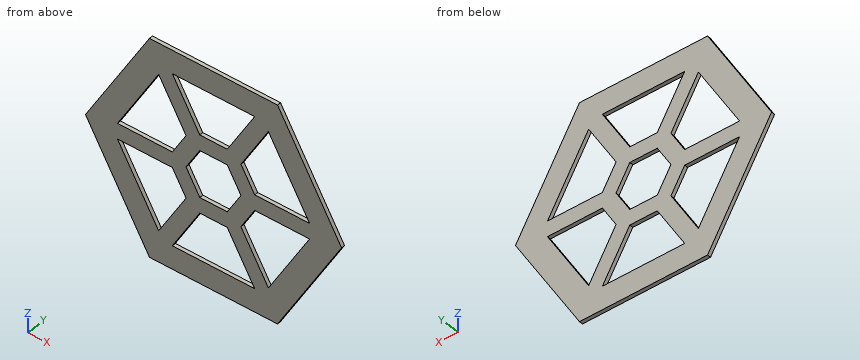
Autodesk Inventor part; units mm, degrees
ref_plane "YZ Plane" through (0, 0, 0) normal (1, 0, 0) x (0, 1, 0)
ref_plane "XZ Plane" through (0, 0, 0) normal (0, 1, 0) x (-1, 0, 0)
ref_plane "XY Plane" through (0, 0, 0) normal (0, 0, 1) x (1, 0, 0)
sketch "Sketch6" plane through (0, 0, 0) normal (0, 1, 0) x (-1, 0, 0)
  circle A0 centre (32.5, -48.5) radius 70
  line L0 (102.5, -48.5) -> (67.5, -109.1218)
  line L1 (67.5, -109.1218) -> (-2.5, -109.1218)
  line L2 (-2.5, -109.1218) -> (-37.5, -48.5)
  line L3 (-37.5, -48.5) -> (-2.5, 12.1218)
  line L4 (-2.5, 12.1218) -> (67.5, 12.1218)
  line L5 (67.5, 12.1218) -> (102.5, -48.5)
  line L6 (32.5, 12.1218) -> (47.5, 12.1218)
  line L7 (47.5, 12.1218) -> (47.5, 5.6218)
  line L8 (47.5, 5.6218) -> (17.5, 5.6218)
  line L9 (17.5, 5.6218) -> (17.5, 12.1218)
  line L10 (47.5, 5.6218) -> (56.6924, 5.6218) construction
  line L11 (17.5, 8.8718) -> (20, 8.8718)
  line L12 (47.5, 8.8718) -> (45, 8.8718)
  line L13 (45, 8.8718) -> (45, 10.1218)
  line L14 (45, 10.1218) -> (20, 10.1218)
  line L15 (20, 10.1218) -> (20, 7.6218)
  line L16 (20, 7.6218) -> (45, 7.6218)
  line L17 (45, 7.6218) -> (45, 10.1218)
  line L18 (47.5, 5.6218) -> (56.6924, 5.6218)
  line L19 (17.5, 5.6218) -> (11, 5.6218)
  line L20 (17.5, 12.1218) -> (11, 5.6218)
  line L21 (17.5, 12.1218) -> (26.6924, 12.1218) construction
  line L22 (47.5, 12.1218) -> (54, 5.6218)
  line L23 (85, -18.1891) -> (77.5, -5.1987)
  line L24 (77.5, -5.1987) -> (71.8708, -8.4487)
  line L25 (71.8708, -8.4487) -> (86.8708, -34.4295)
  line L26 (86.8708, -34.4295) -> (92.5, -31.1795)
  line L27 (71.8708, -8.4487) -> (67.2746, -0.4879) construction
  line L28 (89.6854, -32.8045) -> (88.4354, -30.6394)
  line L29 (74.6854, -6.8237) -> (75.9354, -8.9888)
  line L30 (75.9354, -8.9888) -> (77.0179, -8.3638)
  line L31 (77.0179, -8.3638) -> (89.5179, -30.0144)
  line L32 (89.5179, -30.0144) -> (87.3529, -31.2644)
  line L33 (87.3529, -31.2644) -> (74.8529, -9.6138)
  line L34 (74.8529, -9.6138) -> (77.0179, -8.3638)
  line L35 (71.8708, -8.4487) -> (67.2746, -0.4879)
  line L36 (86.8708, -34.4295) -> (90.1208, -40.0587)
  line L37 (92.5, -31.1795) -> (90.1208, -40.0587)
  line L38 (92.5, -31.1795) -> (87.9038, -23.2187) construction
  line L39 (77.5, -5.1987) -> (68.6208, -2.8196)
  line L40 (71.8708, -88.5513) -> (67.2746, -96.5121) construction
  line L41 (74.6854, -90.1763) -> (75.9354, -88.0112)
  line L42 (74.8529, -87.3862) -> (77.0179, -88.6362)
  line L43 (77.5, -91.8013) -> (71.8708, -88.5513)
  line L44 (77.5, -91.8013) -> (68.6208, -94.1804)
  line L45 (71.8708, -88.5513) -> (67.2746, -96.5121)
  line L46 (77.0179, -88.6362) -> (89.5179, -66.9856)
  line L47 (87.3529, -65.7356) -> (74.8529, -87.3862)
  line L48 (71.8708, -88.5513) -> (86.8708, -62.5705)
  line L49 (89.5179, -66.9856) -> (87.3529, -65.7356)
  line L50 (89.6854, -64.1955) -> (88.4354, -66.3606)
  line L51 (86.8708, -62.5705) -> (92.5, -65.8205)
  line L52 (86.8708, -62.5705) -> (90.1208, -56.9413)
  line L53 (92.5, -65.8205) -> (90.1208, -56.9413)
  line L54 (94.9944, -48.5) -> (63.7472, -102.6218)
  line L55 (63.7472, -102.6218) -> (1.2528, -102.6218)
  line L56 (1.2528, -102.6218) -> (-29.9944, -48.5)
  line L57 (-29.9944, -48.5) -> (1.2528, 5.6218)
  line L58 (1.2528, 5.6218) -> (63.7472, 5.6218)
  line L59 (63.7472, 5.6218) -> (94.9944, -48.5)
  line L60 (74.8529, -87.3862) -> (73.1208, -86.3862)
  line L61 (87.3529, -65.7356) -> (85.6208, -64.7356)
  line L62 (87.3529, -31.2644) -> (85.6208, -32.2644)
  line L63 (74.8529, -9.6138) -> (73.1208, -10.6138)
  line L64 (45, 7.6218) -> (45, 5.6218)
  line L65 (20, 7.6218) -> (20, 5.6218)
  line L66 (-29.9944, -48.5) -> (-22.9944, -48.5)
  line L67 (-29.9944, -48.5) -> (-28.2944, -48.5)
  line L68 (-28.2944, -48.5) -> (-22.9944, -48.5)
  circle A1 centre (-26.9944, -48.5) radius 1.5
  line L69 (-29.9944, -48.5) -> (-23.9944, -48.5)
  line L70 (-23.9944, -48.5) -> (-26.9944, -53.6962)
  line L71 (-23.9944, -48.5) -> (-26.9944, -43.3038)
  point P0 (-27.5473, -52.7386)
  point P1 (-28.2775, -45.5261)
  point P2 (88.4354, -30.6394)
  point P3 (75.9354, -8.9888)
  point P4 (76.4767, -8.6763)
  point P5 (89.6854, -32.8045)
  point P6 (86.4869, -65.2356)
  point P7 (88.4354, -66.3606)
  dimension "d127" = 140
  dimension "d87" = 15
  dimension "d88" = 6.5
  dimension "d91" = 2.5
  dimension "d92" = 2.5
  dimension "d95" = 1.25
  dimension "d96" = 25
  dimension "d97" = 2.5
  dimension "d98" = 25
  dimension "d99" = 135
  dimension "d100" = 0
  dimension "d114" = 1.7
  dimension "d117" = 3
  dimension "d121" = 3
  dimension "d123" = 6
  dimension "d128" = 5.1962
  dimension "d129" = 5.1962
  dimension "d130" = 3
extrude "Fronte" add sketch "Sketch6" along normal blind 2 contours L0 L53 L54 L59 L37 L5 | L5 L39 L35 L59 L58 L18 L22 L4 | L1 L2 L3 L4 L20 L58 L57 L56 L55 L54 L45 L44 L0 | L0 L43 L41 L42 L46 L49 L50 L51 | L51 L52 L53 | L26 L28 L32 L31 L30 L29 L24 L5 | L37 L36 L26 | L7 L12 L13 L14 L15 L11 L9 L4 | L22 L18 L7 | L24 L35 L39 | L44 L45 L43 | L50 L49 L61 L48 L51 | L52 L48 L45 L54 L55 L56 L70 L71 L57 L58 L19 L8 L18 L59 L35 L25 L36 | L26 L25 L62 L32 L28 | L9 L19 L20 | L7 L8 L64 L17 L12 | L29 L34 L63 L25 L24 | L43 L48 L60 L42 L41 | L49 L46 L42 L47 | L32 L33 L34 L30 L31 | L11 L15 L65 L8 L9 | L17 L16 L15 L14 L13 | L47 L60 L48 L61 | L25 L63 L33 L62 | L8 L65 L16 L64 | L71 L66 A1 L57 | L66 A1 L70 L56 | A1 L66 | L66 A1
sketch "Sketch11" plane through (0, 0, 0) normal (0, -1, 0) x (1, 0, 0)
  line L0 (-63.7472, 5.6218) -> (-1.2528, -102.6218)
  line L1 (-94.9944, -48.5) -> (29.9944, -48.5)
  line L2 (-63.7472, -102.6218) -> (-1.2528, 5.6218)
  line L3 (-1.2528, 5.6218) -> (-1.2528, -102.6218)
  circle A0 centre (-32.5, -48.5) radius 55
  line L4 (-5, -0.8686) -> (22.5, -48.5)
  line L5 (22.5, -48.5) -> (-5, -96.1314)
  line L6 (-5, -96.1314) -> (-60, -96.1314)
  line L7 (-60, -96.1314) -> (-87.5, -48.5)
  line L8 (-87.5, -48.5) -> (-60, -0.8686)
  line L9 (-60, -0.8686) -> (-5, -0.8686)
  circle A1 centre (-32.5, -48.5) radius 25
  circle A2 centre (-32.5, -48.5) radius 15
  line L10 (-25, -35.5096) -> (-17.5, -48.5)
  line L11 (-17.5, -48.5) -> (-25, -61.4904)
  line L12 (-25, -61.4904) -> (-40, -61.4904)
  line L13 (-40, -61.4904) -> (-47.5, -48.5)
  line L14 (-47.5, -48.5) -> (-40, -35.5096)
  line L15 (-40, -35.5096) -> (-25, -35.5096)
  line L16 (-20, -26.8494) -> (-7.5, -48.5)
  line L17 (-7.5, -48.5) -> (-20, -70.1506)
  line L18 (-20, -70.1506) -> (-45, -70.1506)
  line L19 (-45, -70.1506) -> (-57.5, -48.5)
  line L20 (-57.5, -48.5) -> (-45, -26.8494)
  line L21 (-45, -26.8494) -> (-20, -26.8494)
  line L22 (-85, -44.1699) -> (-55, -44.1699)
  line L23 (-85, -52.8301) -> (-55, -52.8301)
  line L24 (-55, -96.1314) -> (-40, -70.1506)
  line L25 (-62.5, -91.8013) -> (-47.5, -65.8205)
  line L26 (-2.5, -91.8013) -> (-17.5, -65.8205)
  line L27 (-10, -96.1314) -> (-25, -70.1506)
  line L28 (20, -44.1699) -> (-10, -44.1699)
  line L29 (20, -52.8301) -> (-10, -52.8301)
  line L30 (-10, -0.8686) -> (-25, -26.8494)
  line L31 (-2.5, -5.1987) -> (-17.5, -31.1795)
  line L32 (-62.5, -5.1987) -> (-47.5, -31.1795)
  line L33 (-55, -0.8686) -> (-40, -26.8494)
  line L34 (-43.75, -42.0048) -> (-51.25, -37.6747)
  line L35 (-70, -52.8301) -> (-70, -44.1699)
  line L36 (2.2476, -108.6846) -> (-67.2476, -108.6846)
  line L37 (-67.2476, -108.6846) -> (-101.9952, -48.5)
  line L38 (-101.9952, -48.5) -> (-67.2476, 11.6846)
  line L39 (-67.2476, 11.6846) -> (2.2476, 11.6846)
  line L40 (2.2476, 11.6846) -> (36.9952, -48.5)
  line L41 (36.9952, -48.5) -> (2.2476, -108.6846)
  point P0 (0, 0)
  point P1 (-62.5, -91.8013)
  point P2 (-47.5, -65.8205)
  point P3 (-10, -96.1314)
  point P4 (-25, -70.1506)
  point P5 (-55, -96.1314)
  point P6 (-10, -52.8301)
  point P7 (-2.5, -91.8013)
  point P8 (20, -52.8301)
  point P9 (20, -44.1699)
  point P10 (-2.5, -5.1987)
  point P11 (-17.5, -31.1795)
  point P12 (-10, -44.1699)
  point P13 (-62.5, -5.1987)
  point P14 (-47.5, -31.1795)
  point P15 (-55, -0.8686)
  point P16 (-40, -26.8494)
  point P17 (-25, -26.8494)
  point P18 (-10, -0.8686)
  dimension "d158" = 110
  dimension "d159" = 50
  dimension "d160" = 30
  dimension "d164" = 360
extrude "Extrusion17" cut sketch "Sketch11" against normal blind 2 contours L32 A1 L22 L8 | L9 L30 A1 L33 | L15 L2 L0 | L0 L1 L14 | A1 L30 L21 L33 | L32 L20 L22 A1 | L4 L3 L28 A1 L31 | L23 A1 L25 L7 | L1 L11 L0 | L2 L13 L1 | L2 L10 L1 | L0 L12 L2 | A1 L28 L16 L31 | L4 L28 L3 | L24 A1 L27 L6 | L5 L3 L29 | L23 L19 L25 A1 | L24 L18 L27 A1 | L26 A1 L29 L3 L5 | L26 L17 L29 A1
properties part number "LightFrontalino" material "Wood (Oak)"
Read the model definition and answer for the solid it produces. Units are mm, in the model's axes. Round coordinates to 2 decimals unless told otherwise and drop trailing zeros. Write each loop counter-clockwise with the first axis right and the second up, starting at its lowest first coordinate (ties: lowest second). Pieces come first, ordered by that corner, then holes. Notation, with made-up numbers: (-38, 45.25) - (1, 45.25) arc R18 ccw to (1, 75.25) - close; hole circle Ø5 at (-18, 16.25). An arc over 180 degrees is marked (long way). Use a Markdown table: item, result.
(1) The part is cut by section B-B (x = -15.5). Write down the section's boundary in (y, z), then the cut area to 3 significant figures.
Reported:
| item | result |
|---|---|
| outline | (0, -109.12) - (2, -109.12) - (2, -96.13) - (0, -96.13) - close; (0, -86.61) - (2, -86.61) - (2, -69.28) - (0, -69.28) - close; (0, -62.36) - (2, -62.36) - (2, -34.64) - (0, -34.64) - close; (0, -27.72) - (2, -27.72) - (2, -10.39) - (0, -10.39) - close; (0, -0.87) - (2, -0.87) - (2, 12.12) - (0, 12.12) - close |
| area | 177 mm2 |
(2) Each of these flat-tipped pins is pushed along its axis until it touches: pin 1 Ø1 at (x, y) = (12, 1.5) entering from +Z; pin 2 Ø1 at (y, z) = (1, -13.5) entering from +X; pin 3 Ø3 at (x, z) = (-82.5, -64) entering from -Y. Where does it stop, or does it pass through?
Reported:
| item | result |
|---|---|
| pin 1 | z = -3.47 |
| pin 2 | x = 17.58 |
| pin 3 | y = 0 |
(3) The part is cut by section C-C (z = -67.5). Write down the section's boundary in (x, y), then the cut area to 3 significant figures.
Reported:
| item | result |
|---|---|
| outline | (-91.53, 0) - (-76.53, 0) - (-76.53, 2) - (-91.53, 2) - close; (-48.47, 0) - (-16.53, 0) - (-16.53, 2) - (-48.47, 2) - close; (11.53, 0) - (26.53, 0) - (26.53, 2) - (11.53, 2) - close |
| area | 124 mm2 |
(4) The part is cut by section A-A (z = -3). Write down the section's boundary in (x, y).
Reported:
| item | result |
|---|---|
| outline | (-76.23, 0) - (-53.77, 0) - (-53.77, 2) - (-76.23, 2) - close; (-11.23, 0) - (11.23, 0) - (11.23, 2) - (-11.23, 2) - close |
(5) The part is cut by section D-D (x = -34). Write down the section's boundary in (y, z), then the cut area to 3 significant figures.
Reported:
| item | result |
|---|---|
| outline | (0, -109.12) - (2, -109.12) - (2, -96.13) - (0, -96.13) - close; (0, -70.15) - (2, -70.15) - (2, -61.49) - (0, -61.49) - close; (0, -35.51) - (2, -35.51) - (2, -26.85) - (0, -26.85) - close; (0, -0.87) - (2, -0.87) - (2, 12.12) - (0, 12.12) - close |
| area | 86.6 mm2 |
(6) Straight lines are drawn through the part: line 1 along Z through (x, y) = (-26.5, 0.8); line 2 along Z through (x, y) = (3, 1.35) (3 decimals); line 3 along X through (y, z) = (0.85, -77.5). For each, find the intervals that lie inside material, in ascending order. Write a range as [from, to].
Reported:
| item | result |
|---|---|
| line 1 | [-109.12, -96.13], [-70.15, -61.49], [-35.51, -26.85], [-0.87, 12.12] |
| line 2 | [-108.256, -82.275], [-52.83, -44.17], [-14.725, 11.256] |
| line 3 | [-85.76, -70.76], [-54.24, -44.24], [-20.76, -10.76], [5.76, 20.76] |
